Solid Edge part; units mm, degrees
sketch "Sketch1" plane through (0, 0, 0) normal (0, -1, 0) x (1, 0, 0)
  line L0 (-38, 0) -> (38, 0)
  line L1 (38, 0) -> (38, 5)
  line L2 (38, 5) -> (-38, 5)
  line L3 (-38, 5) -> (-38, 0)
  dimension "D1" = 38
  dimension "D2" = 38
extrude "Protrusion1" add sketch "Sketch1" against normal blind 62
sketch "Sketch2" plane through (0, 30, 5) normal (0, 0, 1) x (-1, 0, 0)
  circle A0 centre (-12.5, -23) radius 2.2
  circle A1 centre (12.5, -23) radius 2.2
  circle A2 centre (33.5, -23) radius 2.2
  circle A3 centre (-33.5, -23) radius 2.2
extrude "ExtrudedCutout_3" cut sketch "Sketch2" against normal blind 110
sketch "Sketch3" plane through (0, 30, 5) normal (0, 0, 1) x (0, 1, 0)
  line L0 (-30, 22) -> (32, 22)
  line L1 (32, 22) -> (32, 27)
  line L2 (-30, 27) -> (32, 27)
  line L3 (-30, 22) -> (-30, 27)
extrude "ExtrudedProtrusion_4" add sketch "Sketch3" along normal blind 5
mirror "Mirror1" about plane through (0, 0, 0) normal (1, 0, 0) of "ExtrudedProtrusion_4"
sketch "Sketch4" plane through (0, 30, 5) normal (0, 0, 1) x (-1, 0, 0)
  line L0 (38, -13) -> (-38, -13)
  line L1 (-38, -18) -> (-38, -13)
  line L2 (38, -18) -> (-38, -18)
  line L3 (38, -18) -> (38, -13)
extrude "ExtrudedProtrusion_6" add sketch "Sketch4" along normal blind 7
sketch "Sketch5" plane through (0, 21.5, 5) normal (0, 0, 1) x (1, 0, 0)
  line L0 (-14.3036, 16.2021) -> (-11.8036, 13.7021)
  arc A0 (-11.8036, 13.7021) -> (-14.2078, 11.2979) centre (-13.0057, 12.5) cw
  line L1 (-14.2078, 11.2979) -> (-16.7078, 13.7979)
  arc A1 (-16.7078, 13.7979) -> (-14.3036, 16.2021) centre (-15.5057, 15) cw
  line L2 (-14.2078, -12.2979) -> (-16.7078, -14.7979)
  arc A2 (-14.3036, -17.2021) -> (-16.7078, -14.7979) centre (-15.5057, -16) cw
  line L3 (-14.3036, -17.2021) -> (-11.8036, -14.7021)
  arc A3 (-14.2078, -12.2979) -> (-11.8036, -14.7021) centre (-13.0057, -13.5) cw
  line L4 (11.7306, -14.9106) -> (14.3599, -17.2662)
  arc A4 (16.7605, -14.8656) -> (14.3599, -17.2662) centre (15.4943, -16) cw
  line L5 (14.4048, -12.2363) -> (16.7605, -14.8656)
  arc A5 (11.7306, -14.9106) -> (14.4048, -12.2363) centre (12.9943, -13.5) cw
  line L6 (14.2922, 16.2021) -> (11.7922, 13.7021)
  arc A6 (14.1964, 11.2979) -> (11.7922, 13.7021) centre (12.9943, 12.5) cw
  line L7 (14.1964, 11.2979) -> (16.6964, 13.7979)
  arc A7 (14.2922, 16.2021) -> (16.6964, 13.7979) centre (15.4943, 15) cw
  circle A8 centre (-0.0057, -0.5) radius 11.5
  dimension "D1" = 0.0057
extrude "Cutout1" cut sketch "Sketch5" against normal through all
sketch "Sketch6" plane through (32.5, 21.5, 5) normal (0, 0, 1) x (0, -1, 0)
  line L0 (21.5, 5.5) -> (66.5, 5.5)
  line L1 (66.5, 5.5) -> (66.5, -70.5)
  line L2 (66.5, -70.5) -> (21.5, -70.5)
  line L3 (21.5, -70.5) -> (21.5, 5.5)
  dimension "D1" = 21.5
extrude "Protrusion3" add sketch "Sketch6" against normal up to vertex (5 mm away)
sketch "Sketch7" plane through (0, 9.5, 5) normal (0, 0, 1) x (0, -1, 0)
  circle A0 centre (49, -34) radius 1.7
  circle A1 centre (49, 34) radius 1.7
  dimension "D1" = 49
  dimension "D2" = 49
extrude "ExtrudedCutout_9" cut sketch "Sketch7" against normal blind 143.3279
sketch "Sketch8" plane through (0, 19, 0) normal (0, 0, -1) x (0, -1, 0)
  circle A0 centre (58.5, 16) radius 1.7
extrude "ExtrudedCutout_10" cut sketch "Sketch8" against normal blind 316.0197
mirror "Mirror2" about plane through (0, 0, 0) normal (1, 0, 0) of "ExtrudedCutout_10"
sketch "Sketch9" plane through (0, 19, 0) normal (0, 0, -1) x (0, -1, 0)
  circle A0 centre (41.5, 16) radius 1.7
  circle A1 centre (41.5, -16) radius 1.7
  circle A2 centre (41.5, -34) radius 1.7
  circle A3 centre (41.5, 34) radius 1.7
extrude "ExtrudedCutout_11" cut sketch "Sketch9" against normal blind 37.4845
sketch "Sketch10" plane through (0, 55, 5) normal (0, 0, 1) x (0, -1, 0)
  line L0 (-7, 38) -> (7, 38)
  line L1 (7, 38) -> (7, -51.7338)
  line L2 (7, -51.7338) -> (-7, -51.7338)
  line L3 (-7, -51.7338) -> (-7, 38)
extrude "ExtrudedCutout_12" cut sketch "Sketch10" against normal blind 91.7973 and the other way blind 101.9208
sketch "Sketch11" plane through (0, 6.15, 0) normal (0, 0, -1) x (0, -1, 0)
  circle A0 centre (10.15, -33.5) radius 2.2
  circle A1 centre (10.15, 33.5) radius 2.2
  dimension "D1" = 10.15
  dimension "D2" = 10.15
extrude "ExtrudedCutout_13" cut sketch "Sketch11" against normal blind 103.1381
sketch "Sketch12" plane through (0, 6.15, 0) normal (0, 0, -1) x (0, -1, 0)
  line L0 (51.15, 10) -> (51.15, -10)
  line L1 (51.15, -10) -> (38.15, -10)
  arc A0 (33.15, -5) -> (38.15, -10) centre (38.15, -5) ccw
  line L2 (33.15, -5) -> (33.15, 5)
  arc A1 (38.15, 10) -> (33.15, 5) centre (38.15, 5) ccw
  line L3 (38.15, 10) -> (51.15, 10)
extrude "ExtrudedCutout_15" cut sketch "Sketch12" against normal blind 370.0743
sketch "Sketch13" plane through (0, -1, 5) normal (0, 0, 1) x (0, -1, 0)
  line L0 (-1, 27) -> (-1, 22)
  line L1 (-1, 22) -> (8, 22)
  line L2 (8, -22) -> (8, 22)
  line L3 (8, -22) -> (-1, -22)
  line L4 (-1, -22) -> (-1, -27)
  line L5 (-1, -27) -> (8, -27)
  line L6 (8, -37.9639) -> (8, -27)
  line L7 (13, -37.9639) -> (8, -37.9639)
  line L8 (13, -27) -> (13, -37.9639)
  line L9 (13, -27) -> (44, -27)
  line L10 (44, -27) -> (44, -22)
  line L11 (44, -22) -> (13, -22)
  line L12 (13, 22) -> (13, -22)
  line L13 (13, 22) -> (44, 22)
  line L14 (44, 22) -> (44, 27)
  line L15 (44, 27) -> (13, 27)
  line L16 (13, 38) -> (13, 27)
  line L17 (8, 38) -> (13, 38)
  line L18 (8, 27) -> (8, 38)
  line L19 (8, 27) -> (-1, 27)
  dimension "D1" = 1
  dimension "D2" = 8
  dimension "D3" = 13
extrude "ExtrudedProtrusion_8" add sketch "Sketch13" along normal blind 7
sketch "Sketch14" plane through (-24.5, 21.5, 10) normal (0, 0, 1) x (0, -1, 0)
  line L0 (21.5, 51.5) -> (-21.5, 51.5)
  line L1 (-21.5, 46.5) -> (-21.5, 51.5)
  line L2 (-21.5, 46.5) -> (21.5, 46.5)
  line L3 (21.5, 51.5) -> (21.5, 46.5)
  line L4 (21.5, -2.5) -> (-21.5, -2.5)
  line L5 (-21.5, 2.5) -> (-21.5, -2.5)
  line L6 (-21.5, 2.5) -> (21.5, 2.5)
  line L7 (21.5, -2.5) -> (21.5, 2.5)
extrude "ExtrudedProtrusion_9" add sketch "Sketch14" along normal blind 2
sketch "Sketch15" plane through (0, -29.5, 5) normal (0, 0, 1) x (0, -1, 0)
  line L0 (-8.7, -16) -> (-8.7, -18)
  arc A0 (-8.7, -18) -> (-5.3, -18) centre (-7, -18) ccw
  line L1 (-5.3, -16) -> (-5.3, -18)
  line L2 (-5.3, -14) -> (-5.3, -16)
  arc A1 (-8.7, -14) -> (-5.3, -14) centre (-7, -14) cw
  line L3 (-8.7, -14) -> (-8.7, -16)
  line L4 (-8.7, 18) -> (-8.7, 14)
  arc A2 (-8.7, 14) -> (-5.3, 14) centre (-7, 14) ccw
  line L5 (-5.3, 18) -> (-5.3, 14)
  arc A3 (-8.7, 18) -> (-5.3, 18) centre (-7, 18) cw
extrude "ExtrudedCutout_16" cut sketch "Sketch15" against normal blind 2209.1975
mirror "Mirror3" about plane through (24, -36.5, 6) normal (0, -1, 0) of "ExtrudedCutout_16"
mirror "Mirror4" about plane through (24, -31.05, 6) normal (0, -1, 0) of "ExtrudedCutout_16"
sketch "Sketch16" plane through (32.5, 17, 5) normal (0, 0, 1) x (0, -1, 0)
  circle A0 centre (-2.7191, 0.8) radius 1.7
  circle A1 centre (-13.7191, 0.8) radius 1.7
extrude "Cutout4" cut sketch "Sketch16" against normal blind 130.0202
mirror "Mirror5" about plane through (0, 1.5, 6) normal (-1, 0, 0) of "Cutout4"
properties material "ABS Plastic, medium impact"
Geometry: final body of the model. Coordinates: model frame, mm. A direction names the side the tool comes from. Give positions to 0.01 mm unless a question says otherwise; leave off trailing zeros. Write each loop counter-clockwise with the first axis right and the second up, starting at its lowest first coordinate (ties: lowest second). Pieces come first, ordered by that corner, then holes. Notation, with made-up numbers: (-7.75, 33.5) -> (44.25, 33.5) arc R30 ccw to (44.25, 68.5) -> close; hole circle Ø2 at (14, -22). An arc over 180 degrees is marked (long way). Answer as a JSON object with one key per item and string values.
1. Access query for faces 5 (the flat face through (32, -9, 8)), 6 (the flat face through (0, 43, 8)), 7 (the flat face through (-16, -41.3, 3)). Directions: +Z, -Z, +X, -X, +Y, -Y. A direction counts if a zero-diameter tool reaches every point of the face in a straight line with its end or side. Return the directions, or none.
Ans:
{"face 5": "+Z, +X", "face 6": "+Z", "face 7": "+Z, -Z"}
2. Contact query for flat-ended pins moving along their axis: pin 1 (13 mm diameter, centred on x = -11, y = 6, fed in from +Z); pin 2 (5.5 mm diameter, centred on y = 24, z = 8.5, fed in from +X); pin 3 (2 mm diameter, centred on x = -34, y = -22.5, fed in from -Z); pin 4 (3 mm diameter, centred on x = 1.5, z = 2.5, fed in from -Y). Output: stop coordinate, or through.
Ans:
{"pin 1": "stops at z = 5", "pin 2": "stops at x = 27", "pin 3": "passes through", "pin 4": "stops at y = -27"}
3. Ray query, probe 1 along Y at (x, z) = (31, 11); probe 2 along X at (y, z) = (-4, 2); probe 3 along X at (y, z) = (-3.5, 8.5). Return the intervals inside material, ascending. Write a range as from..to.
Ans:
{"probe 1": "y = -14..-9, 43..48", "probe 2": "x = -38..-35.7, -31.3..31.3, 35.7..38", "probe 3": "x = -27..-22, 22..27"}
4. Cut plane B-B on z = 7.75. Output: boundary loops of the cut face in (x, y).
Ans:
{"outline": "(-38, 43) -> (-27, 43) -> (-27, -9) -> (-37.96, -9) -> (-37.96, -14) -> (-27, -14) -> (-27, -45) -> (-22, -45) -> (-22, -14) -> (22, -14) -> (22, -45) -> (27, -45) -> (27, -14) -> (38, -14) -> (38, -9) -> (27, -9) -> (27, 43) -> (38, 43) -> (38, 48) -> (-38, 48) -> close; hole (-22, -9) -> (22, -9) -> (22, 43) -> (-22, 43) -> close"}
5. Cut plane D-D on x = 1. Output: boundary loops of the cut face in (y, z), and give its area (3 significant figures).
Ans:
{"outline": "(-27, 0) -> (9.54, 0) -> (9.54, 5) -> (-9, 5) -> (-9, 12) -> (-14, 12) -> (-14, 5) -> (-27, 5) -> close; (32.46, 0) -> (48, 0) -> (48, 12) -> (43, 12) -> (43, 5) -> (32.46, 5) -> close", "area": "330 mm^2"}
6. Cut plane A-A on y = -22.5. Output: boundary loops of the cut face in (x, z), and give its area (3 significant figures).
Ans:
{"outline": "(-38, 0) -> (-35.7, 0) -> (-35.7, 5) -> (-38, 5) -> close; (-32.3, 0) -> (-19.7, 0) -> (-19.7, 5) -> (-22, 5) -> (-22, 12) -> (-27, 12) -> (-27, 5) -> (-32.3, 5) -> close; (-12.3, 0) -> (12.3, 0) -> (12.3, 5) -> (-12.3, 5) -> close; (19.7, 0) -> (32.3, 0) -> (32.3, 5) -> (27, 5) -> (27, 12) -> (22, 12) -> (22, 5) -> (19.7, 5) -> close; (35.7, 0) -> (38, 0) -> (38, 5) -> (35.7, 5) -> close", "area": "342 mm^2"}
7. Mould query, pull axis Y, two halves, no side actions, for faces 1 (the flat face through (-27, -29, 8)), 2 (the flat face through (-24, -45, 3)), 3 (the flat face through (-16, -20.8, 3)), 4 (the flat face through (-15.44, 7.97, 2.54)). Classes: pulls with the +Y half, pulls with the -Y half, needs draft (parallel to the pull), parting line crosses it, or undercut.
Ans:
{"face 1": "needs draft", "face 2": "pulls with the -Y half", "face 3": "undercut", "face 4": "undercut"}
8. Cut plane C-C on y = -4. Output: boundary loops of the cut face in (x, z).
Ans:
{"outline": "(-38, 0) -> (-35.7, 0) -> (-35.7, 5) -> (-38, 5) -> close; (-31.3, 0) -> (31.3, 0) -> (31.3, 5) -> (27, 5) -> (27, 12) -> (22, 12) -> (22, 5) -> (-22, 5) -> (-22, 12) -> (-27, 12) -> (-27, 5) -> (-31.3, 5) -> close; (35.7, 0) -> (38, 0) -> (38, 5) -> (35.7, 5) -> close"}
